For this review, use the dimensioned drawing (mm, ordinates from the lowest corner) and the shaded views. Coordinates: 2 decimals unless noted, no trailing zeros. Loops run counter-clockwise (first coordinate to the right, second up) from the corner with the lowest first, then second, coordinate; pieces in that order, holes last. Notation, with made-up numbers: M 84.5,43.25 L 105.5,43.25 A13 cw 105.5,52.25 Z; hole C -22.75,33.25 d11. An arc over 180 degrees is marked long. One line per item, written item: value.
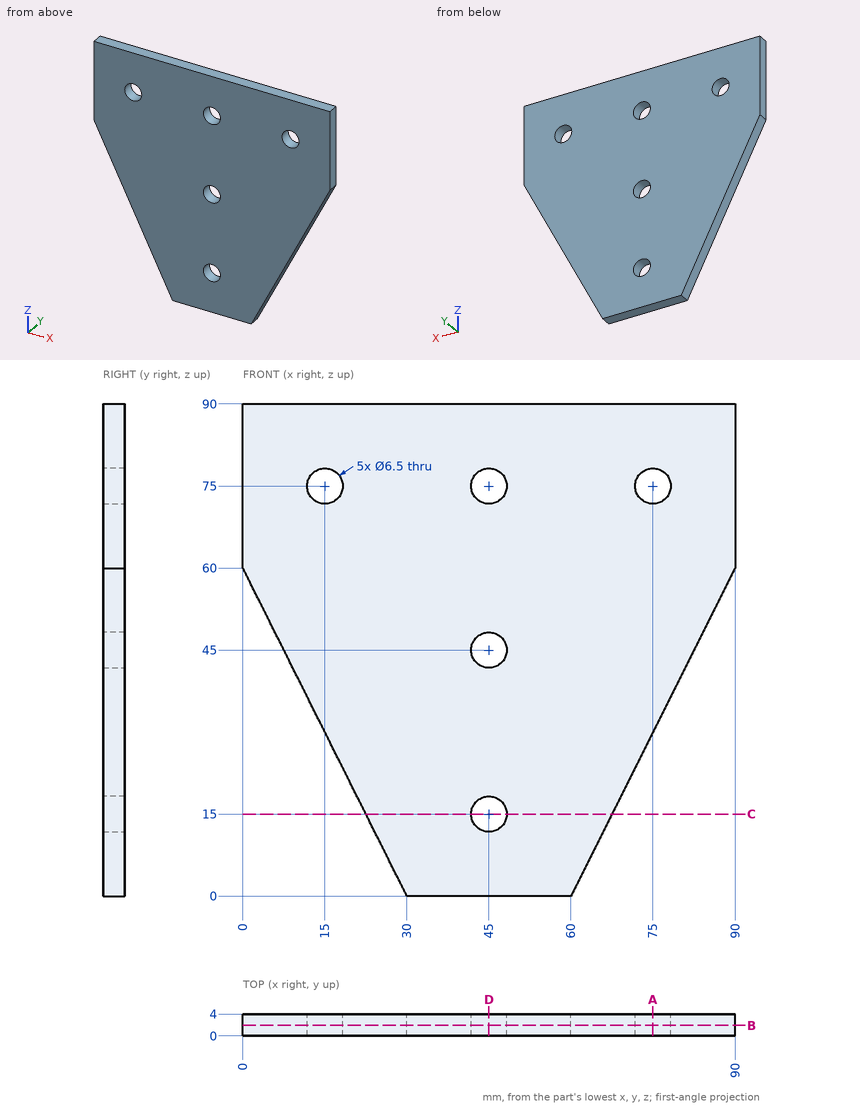
(1) We need section B-B on y = 1.95. State the section outline as (x, z) points, then the cut area to 3 significant figures.
Reply:
outline: M 0,60 L 30,0 L 60,0 L 90,60 L 90,90 L 0,90 Z; hole C 15,75 d6.5; hole C 45,15 d6.5; hole C 45,45 d6.5; hole C 45,75 d6.5; hole C 75,75 d6.5
area: 6,130 mm2
(2) We need section C-C on z = 15. State the section outline as (x, y) points.
Reply:
outline: M 22.5,0 L 41.75,0 L 41.75,4 L 22.5,4 Z; M 48.25,0 L 67.5,0 L 67.5,4 L 48.25,4 Z
(3) We need section A-A on x = 75. State the section outline as (y, z) points, then the cut area to 3 significant figures.
Reply:
outline: M 0,30 L 4,30 L 4,71.75 L 0,71.75 Z; M 0,78.25 L 4,78.25 L 4,90 L 0,90 Z
area: 214 mm2
(4) To check wall thickness, follow line 1 along X through (y, z) = (2.95, 75); line 2 along Z through (x, y) = (72.5, 3.1); line 3 along Z through (x, y) = (42, 3.3). State the ranges of each line that lie inside material, in increasing order. Write a range as [from, to].
Reply:
line 1: x = [0, 11.75], [18.25, 41.75], [48.25, 71.75], [78.25, 90]
line 2: z = [25, 72.92], [77.08, 90]
line 3: z = [0, 13.75], [16.25, 43.75], [46.25, 73.75], [76.25, 90]
(5) Insertion check: pin 1 (2 mm diameter, centred on x = 67, y = 2, fed in from -Z); pin 2 (5 mm diameter, centred on x = 15, z = 75, fed in from -Y) (3 decimals). Each pin has a flat end and moves straight along its axis. Give the tip position at first contact, or say it passes through.
Reply:
pin 1: stops at z = 12
pin 2: passes through
(6) We need section D-D on x = 45. State the section outline as (y, z) points, then the cut area to 3 significant figures.
Reply:
outline: M 0,0 L 4,0 L 4,11.75 L 0,11.75 Z; M 0,18.25 L 4,18.25 L 4,41.75 L 0,41.75 Z; M 0,48.25 L 4,48.25 L 4,71.75 L 0,71.75 Z; M 0,78.25 L 4,78.25 L 4,90 L 0,90 Z
area: 282 mm2
